Here's how the part is built. I have some questions about the finished solid (model axes, mm). A direction names the side the tool comes from. Coordinates: 2 decimals unless noted, no trailing zeros. Loops run counter-clockwise (first coordinate to the right, second up) from the corner with the lowest first, then second, coordinate; pieces in that order, holes last.
from build123d import *

# Parameters (mm, degrees)
SKIZZE1_R                       = 29.95
AUFSATZ_LINEAR_AUSTRAGEN1_DEPTH = 10
SKIZZE2_R                       = 32.75
SKIZZE2_R_2                     = 27.45
AUFSATZ_LINEAR_AUSTRAGEN2_DEPTH = 0.8
SKIZZE5_R                       = 2.3
SCHNITT_LINEAR_AUSTRAGEN1_DEPTH = 10
VERRUNDUNG1_R                   = 50
VERRUNDUNG2_R                   = 6
VERRUNDUNG3_R                   = 4
AUFSATZ_LINEAR_AUSTRAGEN3_DEPTH = 8.306468
FILLET1_R                       = 2
CHAMFER1_SIZE                   = 0.5


with BuildPart() as part:
    # Skizze1 → Aufsatz-Linear austragen1 (new body)
    with BuildSketch(Plane.XY):
        with BuildLine():
            Line((-25.605118216, -22.29305769), (-36.396367746, -22.29305769))
            Line((-36.396367746, -22.29305769), (-38.631857121, -14.29305769))
            Line((-38.631857121, -14.29305769), (-30.794658658, -14.29305769))
            ThreePointArc((-30.794658658, -14.29305769), (-33.95, 0), (-30.794658658, 14.29305769))
            Line((-30.794658658, 14.29305769), (-46.822915195, 15.019747505))
            Line((-46.822915195, 15.019747505), (-49.03277701, 22.928035825))
            Line((-49.03277701, 22.928035825), (-52.800545787, 36.411504164))
            Line((-52.800545787, 36.411504164), (-46.058811618, 38.295388553))
            Line((-46.058811618, 38.295388553), (-41.792257863, 23.026950955))
            Line((-41.792257863, 23.026950955), (-25.605118216, 22.29305769))
            ThreePointArc((-25.605118216, 22.29305769), (0, 33.95), (25.605118216, 22.29305769))
            Line((25.605118216, 22.29305769), (41.792257863, 23.026950955))
            Line((41.792257863, 23.026950955), (46.058811618, 38.295388553))
            Line((46.058811618, 38.295388553), (52.800545787, 36.411504164))
            Line((52.800545787, 36.411504164), (49.03277701, 22.928035825))
            Line((49.03277701, 22.928035825), (46.822915195, 15.019747505))
            Line((46.822915195, 15.019747505), (30.794658658, 14.29305769))
            ThreePointArc((30.794658658, 14.29305769), (33.95, 0), (30.794658658, -14.29305769))
            Line((30.794658658, -14.29305769), (38.631857121, -14.29305769))
            Line((38.631857121, -14.29305769), (36.396367746, -22.29305769))
            Line((36.396367746, -22.29305769), (25.605118216, -22.29305769))
            ThreePointArc((25.605118216, -22.29305769), (0, -33.95), (-25.605118216, -22.29305769))
        make_face()
        Circle(SKIZZE1_R, mode=Mode.SUBTRACT)
    extrude(amount=AUFSATZ_LINEAR_AUSTRAGEN1_DEPTH)

    # Skizze2 → Aufsatz-Linear austragen2 (add)
    with BuildSketch(Plane.XY.offset(10)):
        Circle(SKIZZE2_R)
        Circle(SKIZZE2_R_2, mode=Mode.SUBTRACT)
    extrude(amount=-AUFSATZ_LINEAR_AUSTRAGEN2_DEPTH)

    # Skizze5 → Schnitt-Linear austragen1 (cut)
    with BuildSketch(Plane(origin=(32.796772797, -9.164604643, 0), x_dir=(0, 0, 1), z_dir=(-0.9631048813334842, 0.2691263412444341, 0))):
        with Locations(Location((5, 41.61405755, 0), (0, 0, 270))):
            Circle(SKIZZE5_R)
    schnitt_linear_austragen1 = extrude(amount=-SCHNITT_LINEAR_AUSTRAGEN1_DEPTH, mode=Mode.SUBTRACT)

    # Spiegeln1: Schnitt-Linear austragen1 across plane
    add(schnitt_linear_austragen1.mirror(Plane(origin=(0, 0, 0), x_dir=(0, 0, 1), z_dir=(1, 0, 0))), mode=Mode.SUBTRACT)

    # Verrundung1
    # the kernel refuses this fillet: 50 mm, written as the material it adds along each edge
    with BuildSketch(Plane(origin=(-25.605118216, 22.29305769, 0), x_dir=(-0.9989738125947814, 0.045291519623947715, 0), z_dir=(0, 0, 1))) as verrundung1_piece_1:
        with BuildLine():
            CenterArc((18.087510266, -49.964502541), VERRUNDUNG1_R, 92.159120897, 29.993366161)
            Line((-8.521208788, -7.632764208), (-9.053383169, -6.786129441))
            ThreePointArc((-9.053383169, -6.786129441), (-4.604005024, -3.433010053), (-0.783167276, 0.621811079))
            Line((-0.783167276, 0.621811079), (0, 1))
            ThreePointArc((0, 1), (8.101883875, 1), (16.1660929, 0.999290051))
            Line((16.1660929, 0.999290051), (16.20376775, 0))
        make_face()
    extrude(amount=10)
    with BuildSketch(Plane(origin=(25.605118216, 22.29305769, 0), x_dir=(-0.7743254156963487, 0.6327876030760059, 0), z_dir=(0, 0, 1))) as verrundung1_piece_2:
        with BuildLine():
            CenterArc((19.863886687, -49.285246753), VERRUNDUNG1_R, 99.699501479, 29.993366161)
            Line((-12.069715077, -10.811293506), (-12.708387112, -10.041814441))
            ThreePointArc((-12.708387112, -10.041814441), (-6.702066157, -4.660775852), (-0.667208619, 0.744870901))
            Line((-0.667208619, 0.744870901), (0.168480803, 0.985704935))
            ThreePointArc((0.168480803, 0.985704935), (5.719923266, 0.514682545), (11.271365728, 0.985704935))
            Line((11.271365728, 0.985704935), (11.439846531, 0))
        make_face()
    extrude(amount=10)
    with BuildSketch(Plane(origin=(-25.605118216, -22.29305769, 0), x_dir=(-1, 0, 0), z_dir=(0, 0, 1))) as verrundung1_piece_3:
        with BuildLine():
            CenterArc((17.927143088, 49.488170537), VERRUNDUNG1_R, 238.764970405, 23.029881184)
            Line((-8.000350244, 6.735801135), (-8.51890011, 5.880753747))
            ThreePointArc((-8.51890011, 5.880753747), (-4.38330809, 2.912839933), (-0.754200831, -0.65664382))
            Line((-0.754200831, -0.65664382), (0, -1))
            ThreePointArc((0, -1), (5.395624765, -1), (10.648531659, -0.989763411))
            Line((10.648531659, -0.989763411), (10.79124953, 0))
        make_face()
    extrude(amount=10)
    with BuildSketch(Plane(origin=(25.605118216, -22.29305769, 0), x_dir=(-0.7649741312009661, -0.6440610053351523, 0), z_dir=(0, 0, 1))) as verrundung1_piece_4:
        with BuildLine():
            CenterArc((18.15960016, 49.403344062), VERRUNDUNG1_R, 238.109839077, 23.029881184)
            Line((-8.255026734, 6.950223021), (-8.783319272, 6.1011606))
            ThreePointArc((-8.783319272, 6.1011606), (-4.771574372, 2.710137379), (-0.644061005, -0.764974131))
            Line((-0.644061005, -0.764974131), (0.154025447, -0.988066881))
            ThreePointArc((0.154025447, -0.988066881), (5.229163914, -0.594870618), (10.304302381, -0.988066881))
            Line((10.304302381, -0.988066881), (10.458327827, 0))
        make_face()
    extrude(amount=10)

    # Verrundung2
    # the kernel refuses this fillet: 6 mm, written as the material it adds along each edge
    with BuildSketch(Plane(origin=(-30.794658658, -14.29305769, 0), x_dir=(-0.31650196905899364, 0.9485918530020063, 0), z_dir=(0, 0, 1))) as verrundung2_piece_1_section:
        with BuildLine():
            CenterArc((8.297060958, 5.962063603), VERRUNDUNG2_R, 165.796112126, 97.757459861)
            Line((2.480488745, 7.434302612), (2.364157301, 7.463747393))
            ThreePointArc((2.364157301, 7.463747393), (1.12641335, 3.755131543), (-0.113831022, 0.037980236))
            Line((-0.113831022, 0.037980236), (0.0134729, -0.119241272))
            ThreePointArc((0.0134729, -0.119241272), (3.811707977, 0.094656778), (7.609943054, -0.119241272))
            Line((7.609943054, -0.119241272), (7.623415954, 0))
        make_face()
    verrundung2_piece_1 = extrude(amount=10, mode=Mode.PRIVATE)
    verrundung2_piece_1 = split(verrundung2_piece_1, bisect_by=Plane(origin=(-38.694932937, -14.067332385, 5), z_dir=(0.9631048813334845, 0.2691263412444326, 0)), keep=Keep.TOP, mode=Mode.PRIVATE)
    add(verrundung2_piece_1)
    with BuildSketch(Plane(origin=(30.794658658, -14.29305769, 0), x_dir=(1, 0, 0), z_dir=(0, 0, 1))) as verrundung2_piece_2_section:
        with BuildLine():
            CenterArc((8.281601092, 5.983519558), VERRUNDUNG2_R, 167.994917884, 97.757459861)
            Line((2.412826161, 7.231510266), (2.295450662, 7.256470081))
            ThreePointArc((2.295450662, 7.256470081), (1.296203729, 3.585796077), (-0.1088471, 0.050520381))
            Line((-0.1088471, 0.050520381), (0, -0.12))
            ThreePointArc((0, -0.12), (3.918599232, -0.12), (7.828310411, -0.119670391))
            Line((7.828310411, -0.119670391), (7.837198463, 0))
        make_face()
    verrundung2_piece_2 = extrude(amount=10, mode=Mode.PRIVATE)
    verrundung2_piece_2 = split(verrundung2_piece_2, bisect_by=Plane(origin=(38.694932937, -14.067332385, 5), z_dir=(-0.9631048813334845, 0.2691263412444326, 0)), keep=Keep.TOP, mode=Mode.PRIVATE)
    add(verrundung2_piece_2)
    with BuildSketch(Plane(origin=(30.794658658, 14.29305769, 0), x_dir=(0.320743613458383, -0.9471660543039216, 0), z_dir=(0, 0, 1))) as verrundung2_piece_3:
        with BuildLine():
            CenterArc((7.9683768, 5.965018375), VERRUNDUNG2_R, 163.887999515, 99.921963772)
            Line((2.204050499, 7.630113658), (2.088763973, 7.663415564))
            Line((2.088763973, 7.663415564), (-0.115286526, 0.033301906))
            Line((-0.115286526, 0.033301906), (0.012939177, -0.119300368))
            ThreePointArc((0.012939177, -0.119300368), (3.660708963, 0.077937694), (7.308478748, -0.119300368))
            Line((7.308478748, -0.119300368), (7.321417925, 0))
        make_face()
    extrude(amount=10)
    with BuildSketch(Plane(origin=(-30.794658658, 14.29305769, 0), x_dir=(-0.9989738125947842, 0.045291519623885015, 0), z_dir=(0, 0, 1))) as verrundung2_piece_4:
        with BuildLine():
            CenterArc((7.942069821, 6), VERRUNDUNG2_R, 170.078036228, 99.921963772)
            Line((2.031809742, 7.033840317), (1.91360454, 7.054517124))
            ThreePointArc((1.91360454, 7.054517124), (1.090781254, 3.495291211), (-0.111023547, 0.045538687))
            Line((-0.111023547, 0.045538687), (0, -0.12))
            Line((0, -0.12), (7.942069821, -0.12))
            Line((7.942069821, -0.12), (7.942069821, 0))
        make_face()
    extrude(amount=10)

    # Verrundung3
    verrundung3_edges = [part.edges().sort_by_distance(p)[0] for p in [
        (41.792257863, 23.026950955, 5),
        (46.058811618, 38.295388553, 5),
        (46.822915195, 15.019747505, 5),
        (-46.822915195, 15.019747505, 5),
        (-46.058811618, 38.295388553, 5),
        (-41.792257863, 23.026950955, 5),
    ]]
    fillet(verrundung3_edges, radius=VERRUNDUNG3_R)

    # Skizze6 → Aufsatz-Linear austragen3 (add)
    with BuildSketch(Plane(origin=(3.142139221, -11.244568658, 0), x_dir=(0, 0, -1), z_dir=(-0.26912634124443263, 0.9631048813334845, 0))):
        Polygon((-8.5, 41.05316849), (-7.75, 41.80316849), (-2.25, 41.80316849), (-1.5, 41.05316849), align=None)
    aufsatz_linear_austragen3 = extrude(amount=AUFSATZ_LINEAR_AUSTRAGEN3_DEPTH)

    # Mirror1: Aufsatz-Linear austragen3 across plane
    add(aufsatz_linear_austragen3.mirror(Plane(origin=(0, 0, 0), x_dir=(0, 0, 1), z_dir=(1, 0, 0))))

    # Fillet1
    fillet1_edges = [part.edges().sort_by_distance(p)[0] for p in [
        (52.800545787, 36.411504164, 5),
        (-52.800545787, 36.411504164, 5),
    ]]
    fillet(fillet1_edges, radius=FILLET1_R)

    # Chamfer1
    chamfer1_edges = [part.edges().sort_by_distance(p)[0] for p in [
        (-33.949660085, 0.151921409, 0),
        (-33.949660085, 0.151921409, 10),
        (33.949660085, 0.151921409, 0),
        (33.949660085, 0.151921409, 10),
        (41.329691449, 14.77069548, 0),
        (41.329691449, 14.77069548, 10),
        (-34.27649539, -11.909852297, 0),
        (-34.27649539, -11.909852297, 10),
        (34.27649539, -11.909852297, 0),
        (34.27649539, -11.909852297, 10),
        (34.236583606, 12.306764188, 0),
        (34.236583606, 12.306764188, 10),
        (-34.236583606, 12.306764188, 0),
        (-34.236583606, 12.306764188, 10),
        (-41.329691449, 14.77069548, 0),
        (-41.329691449, 14.77069548, 10),
        (43.806086505, 30.233708145, 0),
        (49.932175512, 26.146654573, 0),
        (-50.392783584, 37.084320017, 0),
        (-43.806086505, 30.233708145, 0),
        (-27.277805641, 25.064576342, 0),
        (-46.871858051, 36.851739876, 0),
        (46.871858051, 36.851739876, 0),
        (46.239249313, 15.753731476, 0),
        (-46.239249313, 15.753731476, 0),
        (43.806086505, 30.233708145, 10),
        (27.277805641, 25.064576342, 10),
        (-43.806086505, 30.233708145, 10),
        (-50.392783584, 37.084320017, 10),
        (49.932175512, 26.146654573, 10),
        (-46.871858051, 36.851739876, 10),
        (46.871858051, 36.851739876, 10),
        (46.239249313, 15.753731476, 10),
        (-46.239249313, 15.753731476, 10),
        (41.103257504, 23.846631411, 0),
        (41.103257504, 23.846631411, 10),
        (-41.103257504, 23.846631411, 0),
        (-41.103257504, 23.846631411, 10),
        (-49.932175512, 26.146654573, 0),
        (-49.932175512, 26.146654573, 10),
        (50.392783584, 37.084320017, 0),
        (52.078721449, 36.004980947, 0),
        (-52.078721449, 36.004980947, 0),
        (50.392783584, 37.084320017, 10),
        (52.078721449, 36.004980947, 10),
        (-52.078721449, 36.004980947, 10),
        (37.514112433, -18.29305769, 0),
        (-37.514112433, -18.29305769, 0),
        (-37.514112433, -18.29305769, 10),
        (37.514112433, -18.29305769, 10),
        (-29.95, 0, 0),
        (0, -33.95, 0),
        (0, -33.95, 10),
        (0, 33.95, 0),
        (0, 33.95, 10),
        (-26.660994535, -24.713613484, 0),
        (-26.660994535, -24.713613484, 10),
        (26.660994535, -24.713613484, 0),
        (26.660994535, -24.713613484, 10),
        (-27.277805641, 25.064576342, 10),
        (27.277805641, 25.064576342, 0),
    ]]
    chamfer(chamfer1_edges, length=CHAMFER1_SIZE)


solid = part.part
Q1. Will these pins go through, and if not, where does the flat tip stop? P1, Ø5, axis at x = 34.5, z = 9, coming from the +Y side; P2, Ø6, axis at y = 24.5, z = 2.5, coming from the +X side; P3, Ø5, axis at x = 21.5, y = 14, coming from the -Z side.
Q2. Suppose I cut it at A-A on x = 0. Write out the boundary of the cut face in (y, z), and give its area (4 significant figures).
Q3. We'd pull the mould along X, two halves only. Please class faces 4 (the cylindrical face through (52.07, 36.02, 5.06)), 5 (the cylindrical face through (28.567, 8.996, 4.789)), 6 (the cylindrical face through (-33.95, 0.05, 4.94)): pulls with the +X half, pulls with the -X half, needs draft (parallel to the pull), parting line crosses it, or undercut.
Q4. For faces 1 (the flat face through (43.267, 28.304, 4.937)), 2 (the flat face through (44.03, 30.11, 9.75)), 3 (the flat face through (-37.5, -18.35, 0.99)), which set-ups out of +Z, -Z, +X, -X, +Y, -Y let a thin tool reach every point of the face, with its end or its side?
Q5. Please list where these lines run through material, in increasing order: probe 1 along Y at (x, z) = (0, 9.4); probe 2 along X at (y, z) = (30, 1); probe 3 along X at (y, z) = (0, 6).
Check values:
1. P1: stops at y = 23.92
1. P2: stops at x = 50.31
1. P3: stops at z = 9.2
2. outline: (-33.95, 0.5) - (-33.45, 0) - (-30.45, 0) - (-29.95, 0.5) - (-29.95, 9.2) - (-27.45, 9.2) - (-27.45, 10) - (-33.45, 10) - (-33.95, 9.5) - close; (27.45, 9.2) - (29.95, 9.2) - (29.95, 0.5) - (30.45, 0) - (33.45, 0) - (33.95, 0.5) - (33.95, 9.5) - (33.45, 10) - (27.45, 10) - close
2. area: 83.25 mm2
3. face 4: pulls with the +X half
3. face 5: undercut
3. face 6: pulls with the -X half
4. face 1: +Z, -Z, +Y
4. face 2: +Z, +Y
4. face 3: -Z, -X, -Y
5. probe 1: y = -33.95 to -27.45, 27.45 to 33.95
5. probe 2: x = -51.01 to -43.74, -15.89 to 15.89, 43.74 to 51.01
5. probe 3: x = -33.95 to -29.95, 29.95 to 33.95
